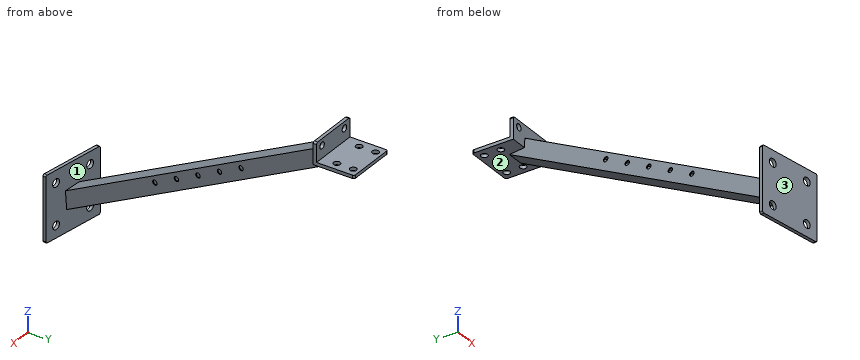
```python
from build123d import *

# Parameters (mm, degrees)
BOSS_EXTRUDE1_DEPTH      = 60
BOSS_EXTRUDE2_DEPTH      = 500
BOSS_EXTRUDE2_DEPTH_BACK = 20
SKETCH3_W                = 20
SKETCH3_H                = 20
SKETCH3_W_2              = 18
SKETCH3_H_2              = 18
CUT_EXTRUDE1_DEPTH       = 60
SKETCH7_W                = 80
SKETCH7_H                = 80
BOSS_EXTRUDE3_DEPTH      = 4
SKETCH8_W                = 96.387466959
SKETCH8_H                = 104.058165024
CUT_EXTRUDE3_DEPTH       = 100
CUT_EXTRUDE4_REACH       = 450.752
SKETCH9_R                = 3.999999996
CUT_EXTRUDE5_REACH       = 450.752
SKETCH10_R               = 4.000000003
CUT_EXTRUDE6_REACH       = 492.61
SKETCH11_R               = 5
FILLET1_R                = 2
FILLET2_R                = 2
SKETCH12_RX              = 3
SKETCH12_RY              = 2.990164225
CUT_EXTRUDE7_DEPTH       = 450.440488821


with BuildPart() as part:
    # Sketch1 → Boss-Extrude1 (new body)
    with BuildSketch(Plane(origin=(0, 0, 0), x_dir=(0, 0, -1), z_dir=(1, 0, 0))):
        Polygon((0, 0), (0, 50), (-4, 50), (-4, 4), (-27, 4), (-27, 0), align=None)
    extrude(amount=BOSS_EXTRUDE1_DEPTH)

    # Sketch3 → Boss-Extrude2 (add, two sides: drawn at the far end of the back side and taken through both)
    with BuildSketch(Plane(origin=(0.734152256, 4.01424851, 2.317627458), x_dir=(0, -0.49999999999998884, 0.866025403784445), z_dir=(-0.1564344650402179, -0.8553631939770945, -0.4938441702975589)).offset(-BOSS_EXTRUDE2_DEPTH_BACK)):
        with Locations((0, -29.630650218)):
            Rectangle(SKETCH3_W, SKETCH3_H)
        with Locations((0, -29.630650218)):
            Rectangle(SKETCH3_W_2, SKETCH3_H_2, mode=Mode.SUBTRACT)
    extrude(amount=BOSS_EXTRUDE2_DEPTH + BOSS_EXTRUDE2_DEPTH_BACK)

    # Sketch5 → Cut-Extrude1 (cut)
    with BuildSketch(Plane.ZY):
        Polygon((4, 4), (4, 36.054903459), (38.781358344, 4), align=None)
    extrude(amount=-CUT_EXTRUDE1_DEPTH, mode=Mode.SUBTRACT)

    # Sketch7 → Boss-Extrude3 (add)
    with BuildSketch(Plane(origin=(-56.75697757, -358.349448921, -6.04e-07), x_dir=(0.9876883403131397, -0.15643446682069614, -2.6345369953248584e-10), z_dir=(0.15643446682069614, 0.9876883403131398, 1.6633811750632153e-09))):
        with Locations((20.602499468, 205.593738915)):
            Rectangle(SKETCH7_W, SKETCH7_H)
    extrude(amount=BOSS_EXTRUDE3_DEPTH)

    # Sketch8 → Cut-Extrude3 (cut)
    with BuildSketch(Plane(origin=(-56.75697757, -358.349448921, -6.04e-07), x_dir=(0.9876883403131398, -0.15643446682069642, -2.6345368640035017e-10), z_dir=(-0.15643446682069642, -0.9876883403131398, -1.6633810921501747e-09))):
        with Locations((22.720042887, -232.311236701)):
            Rectangle(SKETCH8_W, SKETCH8_H)
    extrude(amount=CUT_EXTRUDE3_DEPTH, mode=Mode.SUBTRACT)

    # Sketch9 → Cut-Extrude4 (cut, up to next)
    with BuildSketch(Plane(origin=(0, 0, 0), x_dir=(-1, 0, 0), z_dir=(0, 0, -1)), mode=Mode.PRIVATE) as cut_extrude4_sk1:
        with Locations((-50, 22)):
            Circle(SKETCH9_R)
    cut_extrude4_tool1 = extrude(cut_extrude4_sk1.sketch, amount=-CUT_EXTRUDE4_REACH, mode=Mode.PRIVATE) & part.part
    # Sketch9 → Cut-Extrude4 (cut, up to next)
    with BuildSketch(Plane(origin=(0, 0, 0), x_dir=(-1, 0, 0), z_dir=(0, 0, -1)), mode=Mode.PRIVATE) as cut_extrude4_sk2:
        with Locations((-10, 22)):
            Circle(SKETCH9_R)
    cut_extrude4_tool2 = extrude(cut_extrude4_sk2.sketch, amount=-CUT_EXTRUDE4_REACH, mode=Mode.PRIVATE) & part.part
    # Sketch9 → Cut-Extrude4 (cut, up to next)
    with BuildSketch(Plane(origin=(0, 0, 0), x_dir=(-1, 0, 0), z_dir=(0, 0, -1)), mode=Mode.PRIVATE) as cut_extrude4_sk3:
        with Locations((-10, 42)):
            Circle(SKETCH9_R)
    cut_extrude4_tool3 = extrude(cut_extrude4_sk3.sketch, amount=-CUT_EXTRUDE4_REACH, mode=Mode.PRIVATE) & part.part
    # Sketch9 → Cut-Extrude4 (cut, up to next)
    with BuildSketch(Plane(origin=(0, 0, 0), x_dir=(-1, 0, 0), z_dir=(0, 0, -1)), mode=Mode.PRIVATE) as cut_extrude4_sk4:
        with Locations((-50, 42)):
            Circle(SKETCH9_R)
    cut_extrude4_tool4 = extrude(cut_extrude4_sk4.sketch, amount=-CUT_EXTRUDE4_REACH, mode=Mode.PRIVATE) & part.part
    add(cut_extrude4_tool1.solids().sort_by_distance((50, 22, 0))[0], mode=Mode.SUBTRACT)
    add(cut_extrude4_tool2.solids().sort_by_distance((10, 22, 0))[0], mode=Mode.SUBTRACT)
    add(cut_extrude4_tool3.solids().sort_by_distance((10, 42, 0))[0], mode=Mode.SUBTRACT)
    add(cut_extrude4_tool4.solids().sort_by_distance((50, 42, 0))[0], mode=Mode.SUBTRACT)

    # Sketch10 → Cut-Extrude5 (cut, up to next)
    with BuildSketch(Plane.XZ, mode=Mode.PRIVATE) as cut_extrude5_sk1:
        with Locations(Location((50, 19, 0), (0, 0, 270))):
            Circle(SKETCH10_R)
    cut_extrude5_tool1 = extrude(cut_extrude5_sk1.sketch, amount=-CUT_EXTRUDE5_REACH, mode=Mode.PRIVATE) & part.part
    # Sketch10 → Cut-Extrude5 (cut, up to next)
    with BuildSketch(Plane.XZ, mode=Mode.PRIVATE) as cut_extrude5_sk2:
        with Locations(Location((10, 19, 0), (0, 0, 270))):
            Circle(SKETCH10_R)
    cut_extrude5_tool2 = extrude(cut_extrude5_sk2.sketch, amount=-CUT_EXTRUDE5_REACH, mode=Mode.PRIVATE) & part.part
    add(cut_extrude5_tool1.solids().sort_by_distance((50, 0, 19))[0], mode=Mode.SUBTRACT)
    add(cut_extrude5_tool2.solids().sort_by_distance((10, 0, 19))[0], mode=Mode.SUBTRACT)

    # Sketch11 → Cut-Extrude6 (cut, up to next)
    with BuildSketch(Plane(origin=(-56.75697757, -358.349448921, -6.04e-07), x_dir=(0.9876883403131398, -0.15643446682069645, -2.634536864003504e-10), z_dir=(-0.15643446682069645, -0.9876883403131398, -1.6633810921501756e-09)), mode=Mode.PRIVATE) as cut_extrude6_sk1:
        with Locations((-4.397500532, -180.593738915)):
            Circle(SKETCH11_R)
    cut_extrude6_tool1 = extrude(cut_extrude6_sk1.sketch, amount=-CUT_EXTRUDE6_REACH, mode=Mode.PRIVATE) & part.part
    # Sketch11 → Cut-Extrude6 (cut, up to next)
    with BuildSketch(Plane(origin=(-56.75697757, -358.349448921, -6.04e-07), x_dir=(0.9876883403131398, -0.15643446682069645, -2.634536864003504e-10), z_dir=(-0.15643446682069645, -0.9876883403131398, -1.6633810921501756e-09)), mode=Mode.PRIVATE) as cut_extrude6_sk2:
        with Locations((45.602499468, -180.593738915)):
            Circle(SKETCH11_R)
    cut_extrude6_tool2 = extrude(cut_extrude6_sk2.sketch, amount=-CUT_EXTRUDE6_REACH, mode=Mode.PRIVATE) & part.part
    # Sketch11 → Cut-Extrude6 (cut, up to next)
    with BuildSketch(Plane(origin=(-56.75697757, -358.349448921, -6.04e-07), x_dir=(0.9876883403131398, -0.15643446682069645, -2.634536864003504e-10), z_dir=(-0.15643446682069645, -0.9876883403131398, -1.6633810921501756e-09)), mode=Mode.PRIVATE) as cut_extrude6_sk3:
        with Locations((45.602499468, -230.593738915)):
            Circle(SKETCH11_R)
    cut_extrude6_tool3 = extrude(cut_extrude6_sk3.sketch, amount=-CUT_EXTRUDE6_REACH, mode=Mode.PRIVATE) & part.part
    # Sketch11 → Cut-Extrude6 (cut, up to next)
    with BuildSketch(Plane(origin=(-56.75697757, -358.349448921, -6.04e-07), x_dir=(0.9876883403131398, -0.15643446682069645, -2.634536864003504e-10), z_dir=(-0.15643446682069645, -0.9876883403131398, -1.6633810921501756e-09)), mode=Mode.PRIVATE) as cut_extrude6_sk4:
        with Locations((-4.397500532, -230.593738915)):
            Circle(SKETCH11_R)
    cut_extrude6_tool4 = extrude(cut_extrude6_sk4.sketch, amount=-CUT_EXTRUDE6_REACH, mode=Mode.PRIVATE) & part.part
    add(cut_extrude6_tool1.solids().sort_by_distance((-61.100338, -357.661528, -180.59374))[0], mode=Mode.SUBTRACT)
    add(cut_extrude6_tool2.solids().sort_by_distance((-11.715921, -365.483251, -180.59374))[0], mode=Mode.SUBTRACT)
    add(cut_extrude6_tool3.solids().sort_by_distance((-11.715921, -365.483251, -230.59374))[0], mode=Mode.SUBTRACT)
    add(cut_extrude6_tool4.solids().sort_by_distance((-61.100338, -357.661528, -230.59374))[0], mode=Mode.SUBTRACT)

    # Fillet1
    fillet1_edges = [part.edges().sort_by_distance(p)[0] for p in [
        (60, 50, 2),
        (60, 2, 27),
        (0, 2, 27),
        (0, 50, 2),
    ]]
    fillet(fillet1_edges, radius=FILLET1_R)

    # Fillet2
    # the kernel refuses this fillet: 2 mm, written as the material it takes off along each edge
    with BuildSketch(Plane(origin=(-76.697835011, -360.253452555, -245.593739522), x_dir=(2.0026115353614065e-15, -1.6841157483071222e-09, 1.0), z_dir=(0.15643446682069614, 0.9876883403131398, 1.6633811750632153e-09)), Plane(origin=(-76.697835011, -360.25345269, -165.593739522), x_dir=(0.9876883403131398, -0.15643446682069614, -2.634550355651499e-10), z_dir=(0.15643446682069614, 0.9876883403131398, 1.6633811750632153e-09))) as fillet2_piece_1:
        with BuildLine():
            CenterArc((FILLET2_R, FILLET2_R), FILLET2_R, 180, 90)
            Line((0, FILLET2_R), (0, 0))
            Line((0, 0), (FILLET2_R, 0))
        make_face()
    extrude(amount=14, mode=Mode.SUBTRACT)
    with BuildSketch(Plane(origin=(2.317232214, -372.768210036, -165.593739543), x_dir=(-0.9876883403131398, 0.15643446682069614, 2.634550355651978e-10), z_dir=(0.15643446682069614, 0.9876883403131398, 1.6633811750632153e-09)), Plane(origin=(2.317232214, -372.768209901, -245.593739543), x_dir=(3.518887041216593e-15, -1.6841159884615724e-09, 1.0), z_dir=(0.15643446682069614, 0.9876883403131398, 1.6633811750632153e-09))) as fillet2_piece_2:
        with BuildLine():
            CenterArc((FILLET2_R, -FILLET2_R), FILLET2_R, 90, 90)
            Line((0, -FILLET2_R), (0, 0))
            Line((0, 0), (FILLET2_R, 0))
        make_face()
    extrude(amount=14, mode=Mode.SUBTRACT)

    # Sketch12 → Cut-Extrude7 (cut, through all)
    with BuildSketch(Plane(origin=(19.388964338, -2.659486302, -1.535455133), x_dir=(0.07749165674017042, -0.01062913913579635, 0.9969363392598826), z_dir=(-0.9876883405951398, 0.13547622075225838, 0.0782172325201072))):
        with Locations(Location((-61.225870001, -111.995471629), (0, 0, 75.129892126))):
            Ellipse(SKETCH12_RX, SKETCH12_RY)
        with Locations(Location((-78.507188468, -142.423004822), (0, 0, 75.129892126))):
            Ellipse(SKETCH12_RX, SKETCH12_RY)
        with Locations(Location((-95.788506935, -172.850538016), (0, 0, 75.129892126))):
            Ellipse(SKETCH12_RX, SKETCH12_RY)
        with Locations(Location((-113.069825401, -203.278071209), (0, 0, 75.129892126))):
            Ellipse(SKETCH12_RX, SKETCH12_RY)
        with Locations(Location((-130.351143868, -233.705604403), (0, 0, 75.129892126))):
            Ellipse(SKETCH12_RX, SKETCH12_RY)
    extrude(amount=-CUT_EXTRUDE7_DEPTH, mode=Mode.SUBTRACT)


solid = part.part
```
The model under review builds one solid part; all positions refer to its coordinate system, in mm. Face numbers are marked on the shaded views. Give positions to 0.01 mm unless a question says otherwise; leave off trailing zeros. Loops run counter-clockwise (first coordinate to the right, second up) from the corner with the lowest first, then second, coordinate; pieces in that order, holes last. Notation, with made-up numbers: (30, 7) -> (75, 7) arc R17 cw to (75, 35) -> close; hole circle Ø1 at (-2, -30.5). An arc over 180 degrees is marked (long way). Use CSV: the item, a comma, the result in double quotes.
1. The part is to be moulded in two halves that separate along Y. For the marked faces 1, 2 and 3, say which applies: +Y half, -Y half, draft (parallel to the pull), parting line (faces both ways), or undercut.
Result:
face 1,"undercut"
face 2,"draft"
face 3,"-Y half"
2. To check wall thickness, follow probe 1 along Y at (x, z) = (50, 1.3); probe 2 along X at (y, z) = (1.7, 19); probe 3 along Z at (x, y) = (-23.5, -281.5). State the ranges of each line that lie inside material, in increasing order. Write a range as from..to.
Result:
probe 1,"y = 0..18, 26..38, 46..50"
probe 2,"x = 0..6, 14..46, 54..60"
probe 3,"z = -174.07..-172.92, -152.13..-150.98"
3. Consider section A-A, the plane y = -337. Write out the cut boundary in (x, z), then the cut area to 3 significant figures.
Result:
outline,"(-42.67, -206.11) -> (-22.42, -206.11) -> (-20.59, -183.02) -> (-40.84, -183.02) -> close; hole (-41.57, -204.96) -> (-23.34, -204.96) -> (-21.7, -184.17) -> (-39.92, -184.17) -> close"
area,"88.9 mm²"
4. For P1, Ø11.5, axis at x = 26.5, z = 5, coming from the -Y side; P2, Ø17.5, axis at x = -45, y = -358, coming from the +Z side; P3, Ø6.5, axis at x = 10, y = 22, coming from the -Z side; P4, Ø20, axis at y = 29, z = 12.5, coming from the -X side, all flat-tipped, find the tip position at first contact; note any pin that passes through.
Result:
P1,"stops at y = -21.3"
P2,"stops at z = -165.59"
P3,"passes through"
P4,"stops at x = 0"
5. Consider section C-C, the plane x = -61. Count the separate pieces of the cut face and the enclosed holes in it, then the cut area to 3 significant figures.
Result:
separate pieces,"3"
enclosed holes,"0"
area,"243 mm²"
6. Consider section B-B, the plane x = 29.5. Write out the cut boundary in (y, z).
Result:
outline,"(-63.09, -24.88) -> (-53.09, -42.2) -> (20, 0) -> (50, 0) -> (50, 4) -> (4, 4) -> (4, 27) -> (0, 27) -> (0, 11.55) -> close; hole (-57.06, -22.55) -> (-48.06, -38.14) -> (18, 0) -> (0, 0) -> (0, 10.39) -> close"
